Build history of the part. All positions in model axes, mm. A direction names the side the tool comes from. Give positions to 0.01 mm unless a question says otherwise; leave off trailing zeros. Loops run counter-clockwise (first coordinate to the right, second up) from the corner with the lowest first, then second, coordinate; pieces in that order, holes last. Notation, with made-up numbers: M -6,-4.75 L 1,-4.75 A10 cw 1,-0.75 Z; hole C 43,87 d5. An arc over 180 degrees is marked long. Answer as a JSON object with one key per item and string values. Group by question number.
1. Drill centre lines: line 1 along Y through (x, z) = (23.5, 9); line 2 along X through (y, z) = (8.5, 67); line 3 along Y through (x, z) = (1, 5.5). Where is each one in solid material? Low to high. Write a range as [from, to].
2. Drop flat-ended pins along their axis: pin 1 Ø12.5 at (x, y) = (37, -16.5) entering from +Z; pin 2 Ø7.5 at (x, z) = (0, 16.5) entering from -Y; pin 3 Ø10 at (x, y) = (-8.5, -2) entering from +Z. Give the stop position or say it passes through.
3. Slice it at C-C (z = 18). List the corners of the cut face in (x, y).
4. Slice it at D-D (y = 16). List the corners of the cut face in (x, z), then the cut area to 3 significant figures.
5. 3-axis set-ups, long thin cutter, end or side, ignore diameter. For faces 1 (the face through (1, -7.5, 34)), 2 (the face through (1, 17, 75)), 3 (the face through (0, 2, 35)), 4 (the face through (20, -23, 15)), 5 (the face through (1, 20.5, 5)): which of +Z, -Z, +X, -X, +Y, -Y reach the whole face in a straight line?
6. Slice it at A-A (y = -11). List the corners of the cut face in (x, z), then the cut area to 3 significant figures.
7. Slice it at B-B (x = 39.5). List the corners of the cut face in (y, z), then the cut area to 4 significant figures.
8. Mould opens along Y. For faces 6 (the face through (-35, -32.5, 13)), 7 (the face through (35, -20.5, 5)), 8 (the face through (25, 2, 55)) say: released by +Y, released by -Y, zero draft, split by the parting line, or undercut.
from build123d import *

# Parameters (mm, degrees)
PAD_DEPTH       = 50
SKETCH001_W     = 41
SKETCH001_H     = 16.329009
POCKET_DEPTH    = 100.001
SKETCH002_W     = 51.750069
SKETCH002_H     = 50
POCKET001_DEPTH = 20
SKETCH003_W     = 42.391335
SKETCH003_H     = 40
POCKET002_DEPTH = 25.001


with BuildPart() as part:
    # Sketch → Pad (new body, symmetric)
    with BuildSketch(Plane.YZ):
        Polygon((-32.5, 0), (32.5, 0), (32.5, 75), (-7.5, 75), (-7.5, 25), (-32.5, 25), align=None)
    extrude(amount=PAD_DEPTH, both=True)

    # Sketch001 → Pocket (cut, through all)
    with BuildSketch(Plane.YZ.offset(50)):
        with Locations((0, 1.835495)):
            Rectangle(SKETCH001_W, SKETCH001_H)
    extrude(amount=-POCKET_DEPTH, mode=Mode.SUBTRACT)

    # Sketch002 → Pocket001 (cut)
    with BuildSketch(Plane(origin=(0, -7.5, 0), x_dir=(0, 0, -1), z_dir=(0, -1, 0))):
        with Locations((-60.875034, 0)):
            Rectangle(SKETCH002_W, SKETCH002_H)
    extrude(amount=-POCKET001_DEPTH, mode=Mode.SUBTRACT)

    # Sketch003 → Pocket002 (cut, through all)
    with BuildSketch(Plane(origin=(0, 0, 25), x_dir=(0, -1, 0), z_dir=(0, 0, 1))):
        with Locations((28.695667, 0)):
            Rectangle(SKETCH003_W, SKETCH003_H)
    extrude(amount=-POCKET002_DEPTH, mode=Mode.SUBTRACT)


solid = part.part
Established:
{
 "1": {"line 1": "y = [-32.5, -20.5], [20.5, 32.5]", "line 2": "x = [-50, -25], [25, 50]", "line 3": "y = [20.5, 32.5]"},
 "2": {"pin 1": "stops at z = 25", "pin 2": "stops at y = -7.5", "pin 3": "stops at z = 35"},
 "3": {"outline": "M -50,-32.5 L -20,-32.5 L -20,-7.5 L 20,-7.5 L 20,-32.5 L 50,-32.5 L 50,32.5 L -50,32.5 Z"},
 "4": {"outline": "M -50,10 L 50,10 L 50,75 L -50,75 Z", "area": "6,500 mm^2"},
 "5": {"face 1": "+Z, +X, -X, -Y", "face 2": "+Z, +X, -X, +Y, -Y", "face 3": "+Z, -Y", "face 4": "+Z, -Z, -Y", "face 5": "-Z, +X, -X"},
 "6": {"outline": "M -50,10 L -20,10 L -20,25 L -50,25 Z; M 20,10 L 50,10 L 50,25 L 20,25 Z", "area": "900 mm^2"},
 "7": {"outline": "M -32.5,0 L -20.5,0 L -20.5,10 L 20.5,10 L 20.5,0 L 32.5,0 L 32.5,75 L -7.5,75 L -7.5,25 L -32.5,25 Z", "area": "3,215 mm^2"},
 "8": {"face 6": "released by -Y", "face 7": "undercut", "face 8": "zero draft"}
}
